from build123d import *

# Parameters (mm, degrees)
BOSS_EXTRUDE1_DEPTH = 12.7
SKETCH2_W           = 7.9375
SKETCH2_H           = 58.7375
CUT_EXTRUDE1_DEPTH  = 39.1
FILLET1_R           = 3.175


with BuildPart() as part:
    # Sketch1 → Boss-Extrude1 (new body)
    with BuildSketch(Plane(origin=(0, 0, 0), x_dir=(0, 0, -1), z_dir=(1, 0, 0))):
        Polygon((0, -10.31875), (0, -19.05), (-71.4375, -19.05), (-71.4375, 19.05), (0, 19.05), (0, 10.31875), (-10.31875, 0), align=None)
    extrude(amount=BOSS_EXTRUDE1_DEPTH)

    # Sketch2 → Cut-Extrude1 (cut, through all)
    with BuildSketch(Plane(origin=(0, 19.05, 0), x_dir=(1, 0, 0), z_dir=(0, 1, 0))):
        with Locations((8.73125, -42.06875)):
            Rectangle(SKETCH2_W, SKETCH2_H)
    extrude(amount=-CUT_EXTRUDE1_DEPTH, mode=Mode.SUBTRACT)

    # Fillet1
    fillet1_edges = [part.edges().sort_by_distance(p)[0] for p in [
        (4.7625, 0, 12.7),
    ]]
    fillet(fillet1_edges, radius=FILLET1_R)


solid = part.part
For this review, take the finished solid that the model builds, in its own axes (mm). A direction names the side the tool comes from. Round coordinates to 2 decimals unless told otherwise and drop trailing zeros. Order: outer loops, then holes, each group sorted by start corner. A loop starts at its lowest first (then second) coordinate and runs counter-clockwise, first axis right, second up. Notation, with made-up numbers: M 38,50.5 L 73,50.5 A28 cw 73,88.5 Z; hole C -9.5,3.25 d6. An arc over 180 degrees is marked long. Use a Markdown table: item, result. Add a question column.
Item 1: Add section D-D, the plane z = 59.5. Give the boundary of the cut face in (x, y).
Item 2: Mouldability with a two-part tool opening along Y and no side actions: class faces 1 (the flat face through (3, 19.05, 28)), 2 (the flat face through (6, 15, 0)), 3 (the flat face through (6.26, -5.09, 5.23)) as released by +Y, released by -Y, zero draft, split by the parting line, or undercut.
Item 3: To check wall thickness, follow line 1 along X through (y, z) = (-7.5, 32.5); line 2 along Z through (x, y) = (9.25, 17.5); line 3 along Z through (x, y) = (2.25, 1.5). State the ranges of each line that lie inside material, in increasing order.
Item 4: Tool access review of faces 4 (the flat face through (4.762, 0, 44)), 5 (the flat face through (6.26, 5.23, 5.09)), 6 (the flat face through (0, 0, 35)): name each direction out of +Z, -Z, +X, -X, +Y, -Y from which nothing blocks a thin tool from reaching the whole face with its end or side.
Item 5: Add section B-B, the plane x = 2.75. Give the boundary of the cut face in (y, z), then the cut area to 3 significant figures.
Item 6: Add section A-A, the plane z = 6. Give the boundary of the cut face in (x, y).
Item 7: Insertion check: pin 1 (8 mm diameter, centred on y = -12.5, z = 10.5, fed in from -X); pin 2 (6 mm diameter, centred on y = 12.5, z = 42.5, fed in from +X); pin 3 (5 mm diameter, centred on x = 11.5, y = 4, fed in from +Z). Each pin has a flat end and moves straight along its axis. Give the tip position at first contact, or say it passes through.
Geometry results:
| question | item | result |
|---|---|---|
| 1 | outline | M 0,-19.05 L 4.76,-19.05 L 4.76,19.05 L 0,19.05 Z |
| 2 | face 1 | released by +Y |
| 2 | face 2 | zero draft |
| 2 | face 3 | undercut |
| 3 | line 1 | x = 0 to 4.76 |
| 3 | line 2 | z = 0 to 12.7 |
| 3 | line 3 | z = 8.82 to 71.44 |
| 4 | face 4 | +Z, +X, +Y, -Y |
| 4 | face 5 | -Z, +X, -X |
| 4 | face 6 | +Z, -Z, -X, +Y, -Y |
| 5 | outline | M -19.05,0 L -10.32,0 L 0,10.32 L 10.32,0 L 19.05,0 L 19.05,71.44 L -19.05,71.44 Z |
| 5 | area | 2,620 mm² |
| 6 | outline | M 0,-19.05 L 12.7,-19.05 L 12.7,-4.32 L 0,-4.32 Z; M 0,4.32 L 12.7,4.32 L 12.7,19.05 L 0,19.05 Z |
| 7 | pin 1 | stops at x = 0 |
| 7 | pin 2 | stops at x = 4.76 |
| 7 | pin 3 | stops at z = 12.7 |
